Build history of the part. All positions in model axes, mm. Face numbers are marked on the shaded views. A direction names the side the tool comes from. Round coordinates to 2 decimals unless told otherwise and drop trailing zeros. Loops run counter-clockwise (first coordinate to the right, second up) from the corner with the lowest first, then second, coordinate; pieces in that order, holes last. Notation, with made-up numbers: (59.5, 42.25) - (106.5, 42.25) arc R27 cw to (106.5, 70.25) - close; hole circle Ø6 at (81, 1.25). An arc over 180 degrees is marked (long way). Put each result on its own line as item: value. Start each with the question number.
from build123d import *

# Parameters (mm, degrees)
F0_W          = 60
F0_H          = 12
F0_W_2        = 58
F0_H_2        = 10
F0_R          = 2.75
F1_DEPTH      = 5
F3_DEPTH      = 30
F3_DEPTH_BACK = 30
F4_START      = 5
F4_DEPTH      = 10.001
F5_R          = 2


with BuildPart() as f1:
    # F0 (on Top) → F1 (new body)
    with BuildSketch(Plane.XY):
        Rectangle(F0_W, F0_H)
        Rectangle(F0_W_2, F0_H_2, mode=Mode.SUBTRACT)
        Rectangle(F0_W_2, F0_H_2)
        with Locations((-20, 0)):
            Circle(F0_R, mode=Mode.SUBTRACT)
        Circle(F0_R, mode=Mode.SUBTRACT)
        with Locations((20, 0)):
            Circle(F0_R, mode=Mode.SUBTRACT)
    extrude(amount=F1_DEPTH)

    # F2 (on Right) → F3 (join, two sides)
    with BuildSketch(Plane.YZ) as f3_sk:
        Polygon((6, 15), (-6, 5), (6, 5), align=None)
    extrude(amount=-F3_DEPTH)
    extrude(f3_sk.sketch, amount=F3_DEPTH_BACK)

    # F0 (on Top) → F4 (cut)
    with BuildSketch(Plane.XY.offset(F4_START)):
        Rectangle(F0_W_2, F0_H_2)
        with Locations((-20, 0)):
            Circle(F0_R, mode=Mode.SUBTRACT)
        Circle(F0_R, mode=Mode.SUBTRACT)
        with Locations((20, 0)):
            Circle(F0_R, mode=Mode.SUBTRACT)
        Circle(F0_R)
        with Locations((-20, 0)):
            Circle(F0_R)
        with Locations((20, 0)):
            Circle(F0_R)
    extrude(amount=F4_DEPTH, mode=Mode.SUBTRACT)

    # F5
    f5_edges = [f1.edges().sort_by_distance(p)[0] for p in [
        (0, 6, 0),
        (30, 0, 0),
        (0, -6, 0),
        (-30, 0, 0),
    ]]
    fillet(f5_edges, radius=F5_R)


solid = f1.part
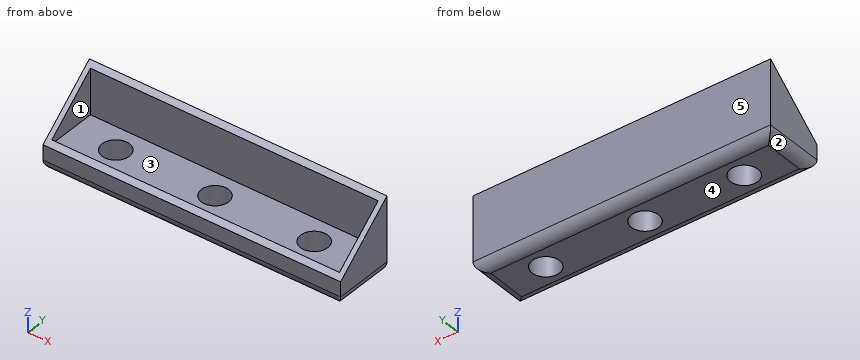
Item 1: Slice it at A-A (x = 0). Give the cut face in (y, z), plus the area to 3 significant figures.
Item 2: Two-plate mould, pull along Y, no slides. Class the marked faces 3, 4 and 5: pulls with the +Y half, pulls with the -Y half, needs draft (parallel to the pull), parting line crosses it, or undercut.
Item 3: Which spindle directions (+Z, -Z, +X, -X, +Y, -Y) get a long thin tool onto all of the face, cutting with end or side? Do the marked faces 1 and 2. Say none if no direction does.
Item 4: Drill centre lines: probe 1 along X at (y, z) = (0, 9.5); probe 2 along X at (y, z) = (0.5, 2.5); probe 3 along Y at (x, z) = (11.5, 11.25). Where is each one in solid material? Low to high. Write a range as [from, to].
Item 5: Slice it at C-C (x = -9). Give the cut face in (y, z).
Item 6: Slice it at B-B (y = 0). Give the cut face in (x, z), plus the area to 3 significant figures.
Item 7: Drop flat-ended pins along their axis: pin 1 Ø3 at (x, y) = (-3, 1.5) entering from +Z; pin 2 Ø2.5 at (x, z) = (-6.5, 8.5) entering from -Y; pin 3 Ø6 at (x, y) = (-2, 2.5) entering from +Z. Give the stop position or say it passes through.
Item 8: Slice it at D-D (z = 10.75). Give the cut face in (x, y), plus the area to 3 significant figures.
Computed values:
1. outline: (-6, 2) arc R2 ccw to (-4, 0) - (-2.75, 0) - (-2.75, 5) - (-5, 5) - (-5, 5.83) - (-6, 5) - close; (2.75, 0) - (4, 0) arc R2 ccw to (6, 2) - (6, 15) - (5, 14.17) - (5, 5) - (2.75, 5) - close
1. area: 40.8 mm^2
2. face 3: undercut
2. face 4: needs draft
2. face 5: pulls with the +Y half
3. face 1: +Z
3. face 2: -Z, -X, +Y, -Y
4. probe 1: x = [-30, -29], [29, 30]
4. probe 2: x = [-30, -22.7], [-17.3, -2.7], [2.7, 17.3], [22.7, 30]
4. probe 3: y = [5, 6]
5. outline: (-6, 2) arc R2 ccw to (-4, 0) - (4, 0) arc R2 ccw to (6, 2) - (6, 15) - (5, 14.17) - (5, 5) - (-5, 5) - (-5, 5.83) - (-6, 5) - close
6. outline: (-30, 2) arc R2 ccw to (-28, 0) - (-22.75, 0) - (-22.75, 5) - (-29, 5) - (-29, 10) - (-30, 10) - close; (-17.25, 0) - (-2.75, 0) - (-2.75, 5) - (-17.25, 5) - close; (2.75, 0) - (17.25, 0) - (17.25, 5) - (2.75, 5) - close; (22.75, 0) - (28, 0) arc R2 ccw to (30, 2) - (30, 10) - (29, 10) - (29, 5) - (22.75, 5) - close
6. area: 226 mm^2
7. pin 1: stops at z = 5
7. pin 2: stops at y = 5
7. pin 3: stops at z = 14.58
8. outline: (-30, 0.9) - (-29, 0.9) - (-29, 5) - (29, 5) - (29, 0.9) - (30, 0.9) - (30, 6) - (-30, 6) - close
8. area: 68.2 mm^2
